Model file for the job. Use its own axes, mm. A direction names the side the tool comes from. Give positions to 0.01 mm unless a question says otherwise; leave off trailing zeros. Loops run counter-clockwise (first coordinate to the right, second up) from the corner with the lowest first, then second, coordinate; pieces in that order, holes last. Notation, with made-up numbers: M 17.5,13 L 34.5,13 A31 cw 34.5,50 Z; hole C -8.5,-12.5 d9. An arc over 180 degrees is marked long. Answer in a Markdown table with one row per item.
```python
from build123d import *

# Parameters (mm, degrees)
SKETCH_R        = 13.5
SKETCH_R_2      = 1.75
SKETCH_R_3      = 4
PAD_DEPTH       = 4
SKETCH001_W     = 3
SKETCH001_H     = 4
SKETCH001_H_2   = 20
PAD001_DEPTH    = 11.5
FILLET_R        = 1.9
FILLET001_R     = 1.9
FILLET002_R     = 1.9
POCKET_DEPTH    = 5
FILLET003_R     = 2
FILLET004_R     = 1.9
FILLET005_R     = 2
SKETCH003_R     = 0.75
POCKET001_DEPTH = 5
SKETCH004_R     = 0.75
POCKET002_DEPTH = 5


with BuildPart() as part:
    # Sketch → Pad (new body)
    with BuildSketch(Plane.XY):
        Circle(SKETCH_R)
        with Locations((-5.656854, -5.656854)):
            Circle(SKETCH_R_2, mode=Mode.SUBTRACT)
        with Locations((5.656854, 5.656854)):
            Circle(SKETCH_R_2, mode=Mode.SUBTRACT)
        with Locations((-6.717514, 6.717514)):
            Circle(SKETCH_R_2, mode=Mode.SUBTRACT)
        with Locations((6.717514, -6.717514)):
            Circle(SKETCH_R_2, mode=Mode.SUBTRACT)
        Circle(SKETCH_R_3, mode=Mode.SUBTRACT)
    extrude(amount=PAD_DEPTH)

    # Sketch001 (on Face7 of Pad) → Pad001 (join)
    with BuildSketch(Plane(origin=(0, 0, 0), x_dir=(1, 0, 0), z_dir=(0, 0, -1))):
        with Locations((13, 0)):
            Rectangle(SKETCH001_W, SKETCH001_H)
        with Locations((-13, -8)):
            Rectangle(SKETCH001_W, SKETCH001_H_2)
    extrude(amount=-PAD001_DEPTH)

    # Fillet
    fillet_edges = [part.edges().sort_by_distance(p)[0] for p in [
        (13, 2, 11.5),
    ]]
    fillet(fillet_edges, radius=FILLET_R)

    # Fillet001
    fillet001_edges = [part.edges().sort_by_distance(p)[0] for p in [
        (13, -2, 11.5),
    ]]
    fillet(fillet001_edges, radius=FILLET001_R)

    # Fillet002
    fillet002_edges = [part.edges().sort_by_distance(p)[0] for p in [
        (-13, -2, 11.5),
    ]]
    fillet(fillet002_edges, radius=FILLET002_R)

    # Sketch002 (on Face5 of Fillet002) → Pocket (cut)
    with BuildSketch(Plane(origin=(-14.5, 0, 0), x_dir=(0, -1, 0), z_dir=(-1, 0, 0))):
        Polygon((-18, 11.5), (-18, 4), (-2.008357, 11.5), align=None)
    extrude(amount=-POCKET_DEPTH, mode=Mode.SUBTRACT)

    # Fillet003
    fillet003_edges = [part.edges().sort_by_distance(p)[0] for p in [
        (-13, 18, 4),
    ]]
    fillet(fillet003_edges, radius=FILLET003_R)

    # Fillet004
    fillet004_edges = [part.edges().sort_by_distance(p)[0] for p in [
        (-13, 18, 0),
    ]]
    fillet(fillet004_edges, radius=FILLET004_R)

    # Fillet005
    fillet005_edges = [part.edges().sort_by_distance(p)[0] for p in [
        (-13, 2.008357, 11.5),
    ]]
    fillet(fillet005_edges, radius=FILLET005_R)

    # Sketch003 (on Face13 of Fillet005) → Pocket001 (cut)
    with BuildSketch(Plane(origin=(-14.5, 0, 0), x_dir=(0, -1, 0), z_dir=(-1, 0, 0))):
        with Locations((-16, 2.2)):
            Circle(SKETCH003_R)
        with Locations((0, 9.5)):
            Circle(SKETCH003_R)
    extrude(amount=-POCKET001_DEPTH, mode=Mode.SUBTRACT)

    # Sketch004 (on Face28 of Pocket001) → Pocket002 (cut)
    with BuildSketch(Plane.YZ.offset(14.5)):
        with Locations((0, 9.5)):
            Circle(SKETCH004_R)
    extrude(amount=-POCKET002_DEPTH, mode=Mode.SUBTRACT)


solid = part.part
```
(1) Saw through at B-B, the plane y = -8. Give the cut face in (x, z).
Established:
| item | result |
|---|---|
| outline | M -10.87,0 L 5.53,0 L 5.53,4 L -10.87,4 Z; M 7.91,0 L 10.87,0 L 10.87,4 L 7.91,4 Z |
(2) Wall check: L1, parallel to X at y = 1, z = 5.5; L2, parallel to Y at x = -7, z = 3; L3, parallel to Z at x = -13.6, y = 0. Give the ranges that are in metal, low to high.
Established:
| item | result |
|---|---|
| L1 | x = -14.5 to -11.5, 11.5 to 14.5 |
| L2 | y = -11.54 to -6.78, -4.54 to 4.99, 8.44 to 11.54 |
| L3 | z = 0 to 8.75, 10.25 to 11.5 |
(3) Saw through at A-A, the plane x = 0. Give the cut face in (y, z), and give its area (3 significant figures).
Established:
| item | result |
|---|---|
| outline | M -13.5,0 L -4,0 L -4,4 L -13.5,4 Z; M 4,0 L 13.5,0 L 13.5,4 L 4,4 Z |
| area | 76.0 mm2 |
(4) Which spindle directions (+Z, -Z, +X, -X, +Y, -Y) get a long thin tool onto all of the face, cutting with end or side? Do faces 4 (the flat face through (13, 2, 6)), 5 (the flat face through (-13, -2, 6)), 6 (the cylindrical face through (-12.98, 2, 11.45)). Say none if no direction does.
Established:
| item | result |
|---|---|
| face 4 | +Z, +X, +Y |
| face 5 | +Z, -X, -Y |
| face 6 | +Z, +X, -X, +Y |
(5) Saw through at C-C, the plane x = 6. Give the cut face in (y, z), and give its area (3 significant figures).
Established:
| item | result |
|---|---|
| outline | M -12.09,0 L -8.31,0 L -8.31,4 L -12.09,4 Z; M -5.12,0 L 3.94,0 L 3.94,4 L -5.12,4 Z; M 7.37,0 L 12.09,0 L 12.09,4 L 7.37,4 Z |
| area | 70.2 mm2 |
(6) Mould opens along Y. For faces 1 (the cylindrical face through (13.021, 1.458, 10.929)), 2 (the flat face through (13, -2, 6)), 3 (the cylindrical face through (13.021, -0.098, 10.244)) say: pulls with the +Y half, pulls with the -Y half, needs draft (parallel to the pull), parting line crosses it, or undercut.
Established:
| item | result |
|---|---|
| face 1 | pulls with the +Y half |
| face 2 | pulls with the -Y half |
| face 3 | undercut |
(7) Saw through at D-D, the plane y = 8. Give the cut face in (x, z), and give its area (3 significant figures).
Established:
| item | result |
|---|---|
| outline | M -14.5,0 L -11.5,0 L -11.5,8.69 L -14.5,8.69 Z; M -10.87,0 L -7.91,0 L -7.91,4 L -10.87,4 Z; M -5.53,0 L 10.87,0 L 10.87,4 L -5.53,4 Z |
| area | 104 mm2 |
(8) Flat gauge pins, fed straight in: P1, Ø3.5, axis at x = 13, z = 7, coming from the +Y side; P2, Ø8, axis at x = 6, y = -2.5, coming from the +Z side; P3, Ø1.7, axis at y = 16, z = 2.2, coming from the -X side; P4, Ø5, axis at y = 11, z = 3, coming from the +X side. Where does each tip first touch, or does it go through?
Established:
| item | result |
|---|---|
| P1 | stops at y = 2 |
| P2 | stops at z = 4 |
| P3 | stops at x = -14.5 |
| P4 | stops at x = 10.49 |
